Work out the finished part from the listing and answer in its coordinate system (mm). Face numbers are marked on the shaded views. A direction names the side the tool comes from. Round coordinates to 2 decimals unless told otherwise and drop trailing zeros. Loops run counter-clockwise (first coordinate to the right, second up) from the corner with the lowest first, then second, coordinate; pieces in that order, holes last. Notation, with made-up numbers: (18.5, 72) - (74.5, 72) arc R33 ccw to (74.5, 102) - close; hole circle Ø3 at (-17, 36.25). An arc over 180 degrees is marked (long way). Return JSON: item names as keys, results as strings.
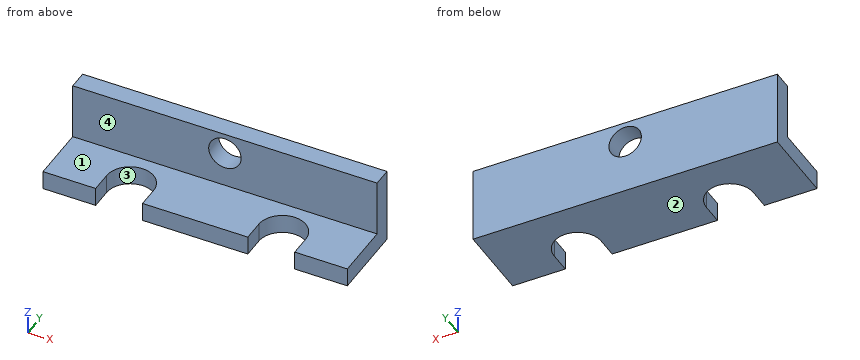
from build123d import *

# Parameters (mm, degrees)
F1_DEPTH = 25.4
F3_DEPTH = 1.5885
F4_R     = 1.35255
F5_DEPTH = 1.5885


with BuildPart() as f1:
    # F0 (on Right) → F1 (new body)
    with BuildSketch(Plane.YZ):
        Polygon((-6.35, 1.5875), (-6.35, 0), (0, 0), (0, 6.35), (-1.5875, 6.35), (-1.5875, 1.5875), align=None)
    extrude(amount=F1_DEPTH)

    # F2 (on face) → F3 (cut, through all)
    with BuildSketch(Plane.XY.offset(1.5875)):
        with BuildLine():
            Line((8.3058, -6.35), (8.3058, -4.5847))
            ThreePointArc((8.3058, -4.5847), (6.35, -2.6289), (4.3942, -4.5847))
            Line((4.3942, -4.5847), (4.3942, -6.35))
            Line((4.3942, -6.35), (8.3058, -6.35))
        make_face()
        with BuildLine():
            ThreePointArc((21.0058, -4.5847), (19.05, -2.6289), (17.0942, -4.5847))
            Line((17.0942, -4.5847), (17.0942, -6.35))
            Line((17.0942, -6.35), (21.0058, -6.35))
            Line((21.0058, -6.35), (21.0058, -4.5847))
        make_face()
    extrude(amount=-F3_DEPTH, mode=Mode.SUBTRACT)

    # F4 (on face) → F5 (cut, through all)
    with BuildSketch(Plane.XZ.offset(1.5875)):
        with Locations((12.7, 4.5847)):
            Circle(F4_R)
    extrude(amount=-F5_DEPTH, mode=Mode.SUBTRACT)


solid = f1.part
1) A flat-ended cylindrical pin translates along its axis: pin 1 (1.4 mm diameter, centred on x = 15, y = -5, fed in from +Z). Find the tip coordinate at first contact, or state that the pin passes through.
Verdict:
{"pin 1": "stops at z = 1.59"}
2) Section D-D (z = 2.75) is taken. Give the vertices of the cut face in (x, y), and give its area (3 significant figures).
Verdict:
{"outline": "(0, -1.59) - (25.4, -1.59) - (25.4, 0) - (0, 0) - close", "area": "40.3 mm2"}
3) Section C-C (x = 2) is taken. Give the vertices of the cut face in (y, z).
Verdict:
{"outline": "(-6.35, 0) - (0, 0) - (0, 6.35) - (-1.59, 6.35) - (-1.59, 1.59) - (-6.35, 1.59) - close"}
4) Section A-A (x = 12.7) is taken. Give the vertices of the cut face in (y, z), and give its area (3 significant figures).
Verdict:
{"outline": "(-6.35, 0) - (0, 0) - (0, 3.23) - (-1.59, 3.23) - (-1.59, 1.59) - (-6.35, 1.59) - close; (-1.59, 5.94) - (0, 5.94) - (0, 6.35) - (-1.59, 6.35) - close", "area": "13.3 mm2"}
5) Find the intervals of material crossed by L1, parallel to Z at x = 12.7, y = -1.2; L2, parallel to X at y = -3.25, z = 0.5; L3, parallel to X at y = -4.75, z = 1, in increasing order.
Verdict:
{"L1": "z = 0 to 3.23, 5.94 to 6.35", "L2": "x = 0 to 4.92, 7.78 to 17.62, 20.48 to 25.4", "L3": "x = 0 to 4.39, 8.31 to 17.09, 21.01 to 25.4"}
6) Section B-B (z = 0.75) is taken. Give the vertices of the cut face in (x, y), and give its area (3 significant figures).
Verdict:
{"outline": "(0, -6.35) - (4.39, -6.35) - (4.39, -4.58) arc R1.96 cw to (8.31, -4.58) - (8.31, -6.35) - (17.09, -6.35) - (17.09, -4.58) arc R1.96 cw to (21.01, -4.58) - (21.01, -6.35) - (25.4, -6.35) - (25.4, 0) - (0, 0) - close", "area": "135 mm2"}
7) A tool of negligible diameter and unlimited length cuts with its end or side. For the marked faces 1 and 2, from which of +Z, -Z, +X, -X, +Y, -Y can it reach the whole face along a straight path? Write none if from no direction.
Verdict:
{"face 1": "+Z, +X, -X, -Y", "face 2": "-Z, +X, -X, +Y, -Y"}
8) Determine the mould class of the marked faces 3 and 4 for opening direction X: pulls with the +X half, pulls with the -X half, needs draft (parallel to the pull), parting line crosses it, or undercut.
Verdict:
{"face 3": "undercut", "face 4": "needs draft"}
